Design review of the part built by this model. Coordinates are the model's own, in mm. A direction names the side the tool comes from. Round coordinates to 2 decimals unless told otherwise and drop trailing zeros. Loops run counter-clockwise (first coordinate to the right, second up) from the corner with the lowest first, then second, coordinate; pieces in that order, holes last. Notation, with made-up numbers: (76, 39) - (94, 39) arc R29 ccw to (94, 70) - close; hole circle Ø11 at (27.5, 4.25). An arc over 180 degrees is marked (long way). One line per question, with ' | ' between items. Start each with the question number.
from build123d import *

# Parameters (mm, degrees)
F0_W        = 36
F0_H        = 33
F1_DEPTH    = 9
F3_DEPTH    = 25
F4_W        = 32
F4_H        = 29
F5_DEPTH    = 2
F6_R        = 0.75
F7_DEPTH    = 4
F8_T1_DEPTH = 48
F8_T3_DEPTH = 51


# Not quite as in the source:
# - a fillet or chamfer that OpenCascade refuses, or shapes differently, is made with other operations: its cross-section is extruded or revolved along the edge and cut away or added


with BuildPart() as f1:
    # F0 (on Front) → F1 (new body)
    with BuildSketch(Plane.XZ):
        with Locations((18, 16.5)):
            Rectangle(F0_W, F0_H)
    extrude(amount=F1_DEPTH)

    # F2 (on face) → F3 (cut)
    with BuildSketch(Plane.XZ.offset(9)):
        with BuildLine():
            ThreePointArc((6.25, 16), (18, 4.25), (29.75, 16))
            ThreePointArc((29.75, 16), (18, 27.75), (6.25, 16))
        make_face()
        with BuildLine():
            ThreePointArc((6.25, 16), (18, 27.75), (29.75, 16))
            Line((29.75, 16), (29.75, 33))
            Line((29.75, 33), (6.25, 33))
            Line((6.25, 33), (6.25, 16))
        make_face()
    extrude(amount=-F3_DEPTH, mode=Mode.SUBTRACT)

    # F4 (on face) → F5 (cut)
    with BuildSketch(Plane.XZ.offset(9)):
        with Locations((18, 16.5)):
            Rectangle(F4_W, F4_H)
    extrude(amount=-F5_DEPTH, mode=Mode.SUBTRACT)

    # F6 (on face) → F7 (cut)
    with BuildSketch(Plane(origin=(0, 0, 0), x_dir=(-1, 0, 0), z_dir=(0, 1, 0))):
        with Locations((-31.5, 30)):
            Circle(F6_R)
        with Locations((-3, 30)):
            Circle(F6_R)
        with Locations((-3, 3)):
            Circle(F6_R)
        with Locations((-31, 3)):
            Circle(F6_R)
    extrude(amount=-F7_DEPTH, mode=Mode.SUBTRACT)

    # F8: fillet of radius 3 on 3 edges, made by hand

    # F8_s2 → F8_t1 (cut)
    with BuildSketch(Plane.XY.offset(-7.5)):
        with BuildLine():
            ThreePointArc((33, -9), (35.1213203436, -8.1213203436), (36, -6))
            Line((36, -6), (36, -9))
            Line((36, -9), (33, -9))
        make_face()
        with BuildLine():
            ThreePointArc((0, -6), (0.8786796564, -8.1213203436), (3, -9))
            Line((3, -9), (0, -9))
            Line((0, -9), (0, -6))
        make_face()
    extrude(amount=F8_T1_DEPTH, mode=Mode.SUBTRACT)

    # F8_s4 → F8_t3 (cut)
    with BuildSketch(Plane.YZ.offset(-7.5)):
        with BuildLine():
            ThreePointArc((-6, 0), (-8.1213203436, 0.8786796564), (-9, 3))
            Line((-9, 3), (-9, 0))
            Line((-9, 0), (-6, 0))
        make_face()
    extrude(amount=F8_T3_DEPTH, mode=Mode.SUBTRACT)


solid = f1.part
1. Machinability: for faces 5 (the face through (33, -4, 33)), 6 (the face through (6.25, -4, 25)), 7 (the face through (19, -7, 4)), 8 (the face through (10, 0, 6)), 9 (the face through (30.785, -1.972, 30.225)), which of the approach directions +Z, -Z, +X, -X, +Y, -Y give a long, thin tool a straight path to every point of the face, cutting with its end or side? Answer none if there is none.
2. Take a section at C-C, the plane z = 3. Give the boundary of the cut face in (x, y), then the cut area to 3 significant figures.
3. Take a section at A-A, the plane z = 30. Give the boundary of the cut face in (x, y).
4. Clearance check with flat-ended pins moving along their axes: P1, Ø1.5, axis at x = 11, y = -6.5, coming from the +Z side; P2, Ø0.8, axis at x = 31.5, z = 30, coming from the +Y side; P3, Ø0.5, axis at x = 24.5, y = -7.5, coming from the +Z side; P4, Ø14.5, axis at x = 18.5, z = 21, coming from the -Y side. State where each tip first meets the part, or that it passes through.
5. Take a section at D-D, the plane x = 18. Give the boundary of the cut face in (y, z), then the cut area to 3 significant figures.
6. The part is to be moulded in two halves that separate along X. For faces 1 (the face through (17.748, -7.711, 0.536)), 2 (the face through (2, -8, 16)), 3 (the face through (4, -8, 31)), 4 (the face through (35.438, -7.748, 16.269)), say which applies: pulls with the +X half, pulls with the -X half, needs draft (parallel to the pull), parting line crosses it, or undercut.
7. Take a section at B-B, the plane y = -2.25. Give the boundary of the cut face in (x, z), then the cut area to 3 significant figures.
8. To check wall thickness, follow line 1 along Z through (x, y) = (3, -0.75); line 2 along X through (y, z) = (-3.75, 16); line 3 along Z through (x, y) = (31.5, -2.5). State the ranges of each line that lie inside material, in increasing order.
Answer list:
1) face 5: +Z, +X, -X, +Y, -Y | face 6: +Z, +Y, -Y | face 7: -Y | face 8: +Z, -Z, +X, -X, +Y | face 9: +Y
2) outline: (0, -6) arc R3 ccw to (2, -8.83) - (2, -7) - (34, -7) - (34, -8.83) arc R3 ccw to (36, -6) - (36, 0) - (31.75, 0) - (31.75, -4) - (30.25, -4) - (30.25, 0) - (3.75, 0) - (3.75, -4) - (2.25, -4) - (2.25, 0) - (0, 0) - close | area: 244 mm²
3) outline: (0, -6) arc R3 ccw to (2, -8.83) - (2, -7) - (6.25, -7) - (6.25, 0) - (3.75, 0) - (3.75, -4) - (2.25, -4) - (2.25, 0) - (0, 0) - close; (29.75, -7) - (34, -7) - (34, -8.83) arc R3 ccw to (36, -6) - (36, 0) - (32.25, 0) - (32.25, -4) - (30.75, -4) - (30.75, 0) - (29.75, 0) - close
4) P1: stops at z = 7.17 | P2: stops at y = -4 | P3: stops at z = 2 | P4: passes through
5) outline: (-8.83, 2) arc R3 ccw to (-6, 0) - (0, 0) - (0, 4.25) - (-7, 4.25) - (-7, 2) - close | area: 31.9 mm²
6) face 1: needs draft | face 2: undercut | face 3: undercut | face 4: pulls with the +X half
7) outline: (0, 0) - (36, 0) - (36, 33) - (29.75, 33) - (29.75, 16) arc R11.75 cw to (6.25, 16) - (6.25, 33) - (0, 33) - close; hole circle Ø1.5 at (3, 3); hole circle Ø1.5 at (3, 30); hole circle Ø1.5 at (31, 3); hole circle Ø1.5 at (31.5, 30) | area: 565 mm²
8) line 1: z = 0 to 2.25, 3.75 to 29.25, 30.75 to 33 | line 2: x = 0 to 6.25, 29.75 to 36 | line 3: z = 0 to 2.44, 3.56 to 29.25, 30.75 to 33
